from build123d import *

# Parameters (mm, degrees)
F0_W     = 86
F0_H     = 10
F1_DEPTH = 12.69
F2_W     = 6.1
F2_H     = 3.7164622918
F4_W     = 6.1
F4_H     = 3.7164622918
F6_R     = 5
F7_R     = 1.5
F8_DEPTH = 10.001


# Not quite as in the source:
# - a feature names something its author has since deleted; it is built from what else it names


with BuildPart() as f1:
    # F0 (on Top) → F1 (new body)
    with BuildSketch(Plane.XY):
        Rectangle(F0_W, F0_H)
    extrude(amount=F1_DEPTH)

    # F2 (on face) → F3 (revolve, cut)
    with BuildSketch(Plane.XZ.offset(5)):
        Polygon((-8.4, 12.69), (-16.5, 12.69), (-16.5, 8.2610268146), (-10.4, 8.2610268146), (-8.4, 8.2610268146), align=None)
        with Locations((-13.45, 6.4027956687)):
            Rectangle(F2_W, F2_H)
        Polygon((-10.4, 4.5445645228), (-16.5, 4.5445645228), (-16.5, 0), (-8.3565199748, 0), (-8.3565199748, 4.5445645228), align=None)
    revolve(axis=Axis((-16.5, -5, 6.345), (0, 0, -1)), mode=Mode.SUBTRACT)

    # F4 (on face) → F5 (revolve, cut)
    with BuildSketch(Plane.XZ.offset(5)):
        Polygon((25.4217400126, 12.69), (17.3217400126, 12.69), (17.3217400126, 8.2610268146), (23.4217400126, 8.2610268146), (25.4217400126, 8.2610268146), align=None)
        with Locations((20.3717400126, 6.4027956687)):
            Rectangle(F4_W, F4_H)
        Polygon((23.4217400126, 4.5445645228), (17.3217400126, 4.5445645228), (17.3217400126, 0), (25.4217400126, 0), (25.4217400126, 4.5445645228), align=None)
    revolve(axis=Axis((17.3217400126, -5, 6.345), (0, 0, -1)), mode=Mode.SUBTRACT)

    # F6
    f6_edges = [f1.edges().sort_by_distance(p)[0] for p in [
        (-43, 0, 12.69),
        (43, 0, 12.69),
    ]]
    fillet(f6_edges, radius=F6_R)

    # F7 (on face) → F8 (cut, through all)
    with BuildSketch(Plane(origin=(0, 5, 0), x_dir=(-1, 0, 0), z_dir=(0, 1, 0))):
        with Locations((-30.9640802443, 6.345)):
            Circle(F7_R)
        with Locations((0, 6.345)):
            Circle(F7_R)
        with Locations((32.0656448603, 6.345)):
            Circle(F7_R)
    extrude(amount=-F8_DEPTH, mode=Mode.SUBTRACT)


solid = f1.part
Check sheet for the modelled part. Datum: model origin and axes. Units: mm. A direction names the side the tool comes from. Give positions to 0.01 mm unless a question says otherwise; leave off trailing zeros. Loops run counter-clockwise (first coordinate to the right, second up) from the corner with the lowest first, then second, coordinate; pieces in that order, holes last. Notation, with made-up numbers: M 21,37 L 75,37 A16 ccw 75,46 Z; hole C 66.25,77 d5. An arc over 180 degrees is marked long. Return JSON: item names as keys, results as strings. Group by question number.
1. Mould release check, pull along X, two halves, no side actions. Record for faces 1 (the flat face through (17.3, 1.4, 4.545)), 2 (the flat face through (43, 0, 4)), 3 (the flat face through (-43, 0, 4)): released by +X, released by -X, zero draft, split by the parting line, or undercut.
2. Tool access check on faces 4 (the flat face through (-1, 5, 5)), 5 (the flat face through (17.4, 1.4, 8.261)), 6 (the cylindrical face through (17.144, 3.098, 2.304)). Record the directions out of +Z, -Z, +X, -X, +Y, -Y that give a thin tool (end or side, any length) a straight path to the whole face; none if there is none.
3. Thickness scan on L1, parallel to X at y = -4.5, z = 2; L2, parallel to X at y = -0.5, z = 7.25; L3, parallel to X at y = -0.5, z = 7.5. Record the ranges inside material, lowest first.
4. Go/stop test with flat-tipped pins: pin 1 (3.5 mm diameter, centred on x = -32.07, z = 6.34, fed in from -Y); pin 2 (4 mm diameter, centred on x = -18.5, y = -1, fed in from +Z); pin 3 (1.8 mm diameter, centred on x = 0, z = 6.345, fed in from -Y). Record where each tip stops, or that it passes through.
5. Cross-section at A-A on y = -3.75. State how many separate pieces and enclosed holes the cut face has, plus the area to 3 significant figures.
6. Cross-section at C-C on x = -16.5. Record the boundary of the cut face in (y, z).
7. Cross-section at D-D on z = 10.25. Record the boundary of the cut face in (x, y), plus the area to 3 significant figures.
8. Cross-section at B-B on x = 0. Record the boundary of the cut face in (y, z) (3 decimals), plus the area to 3 significant figures.
Return value:
{
 "1": {"face 1": "undercut", "face 2": "released by +X", "face 3": "released by -X"},
 "2": {"face 4": "+Z, -Z, +X, -X, +Y", "face 5": "+Z, -Y", "face 6": "-Z, -Y"},
 "3": {"L1": "-43 to -24.63, -8.37 to 9.24, 25.41 to 43", "L2": "-43 to -33.26, -30.87 to -20.62, -12.38 to -1.2, 1.2 to 13.2, 21.44 to 29.77, 32.16 to 43", "L3": "-43 to -33.02, -31.11 to -20.62, -12.38 to -0.96, 0.96 to 13.2, 21.44 to 30.01, 31.92 to 43"},
 "4": {"pin 1": "y = -5", "pin 2": "z = 8.26", "pin 3": "through"},
 "5": {"separate pieces": "3", "enclosed holes": "3", "area": "683 mm^2"},
 "6": {"outline": "M 1.1,4.54 L 3.14,4.54 L 3.14,0 L 5,0 L 5,12.69 L 3.1,12.69 L 3.1,8.26 L 1.1,8.26 Z"},
 "7": {"outline": "M -42.29,-5 L -24.6,-5 A8.1 cw -8.4,-5 L 9.22,-5 A8.1 cw 25.42,-5 L 42.29,-5 L 42.29,5 L -42.29,5 Z", "area": "640 mm^2"},
 "8": {"outline": "M -5,0 L 5,0 L 5,4.845 L -5,4.845 Z; M -5,7.845 L 5,7.845 L 5,12.69 L -5,12.69 Z", "area": "96.9 mm^2"}
}
